from build123d import *

# Parameters (mm, degrees)
F1_DEPTH = 8
F2_W     = 10.1
F2_H     = 10.1
F3_DEPTH = 30
F4_W     = 10.1
F4_H     = 10.1
F5_DEPTH = 33.3550908792
F6_R     = 2


with BuildPart() as f1:
    # F0 (on Right) → F1 (new body, symmetric)
    with BuildSketch(Plane.YZ):
        Polygon((9, -9), (15, -9), (15, 9), (-15, 9), (-15, -9), (-9, -9), (0, -37.9528366029), (16.4139532903, -32.8505531328), align=None)
    extrude(amount=F1_DEPTH, both=True)

    # F2 (on face) → F3 (cut, through all)
    with BuildSketch(Plane(origin=(0, 15, 0), x_dir=(-1, 0, 0), z_dir=(0, 1, 0))):
        Rectangle(F2_W, F2_H)
    extrude(amount=-F3_DEPTH, mode=Mode.SUBTRACT)

    # F4 (on face) → F5 (cut, through all)
    with BuildSketch(Plane(origin=(0, 10.7581183802, -34.608671513), x_dir=(1, 0, 0), z_dir=(0, 0.2968395292, -0.9549273762))):
        with Locations((0, 2.6715557628)):
            Rectangle(F4_W, F4_H)
    extrude(amount=-F5_DEPTH, mode=Mode.SUBTRACT)

    # F6
    f6_edges = [f1.edges().sort_by_distance(p)[0] for p in [
        (0, 15, 9),
        (-8, 0, 9),
        (0, -15, 9),
        (8, 0, 9),
        (-8, 8.206977, -35.401695),
        (-8, 12.706977, -20.925277),
        (-8, 12, -9),
        (-8, 15, 0),
        (-8, -15, 0),
        (-8, -12, -9),
        (-8, -4.5, -23.476418),
        (0, 0, -37.952837),
        (8, -4.5, -23.476418),
        (0, -9, -9),
        (8, 8.206977, -35.401695),
        (8, 12.706977, -20.925277),
        (8, 12, -9),
        (8, 15, 0),
        (8, -15, 0),
        (8, -12, -9),
        (0, 16.413953, -32.850553),
        (0, 9, -9),
        (0, 15, -9),
        (0, -15, -9),
    ]]
    fillet(f6_edges, radius=F6_R)


solid = f1.part
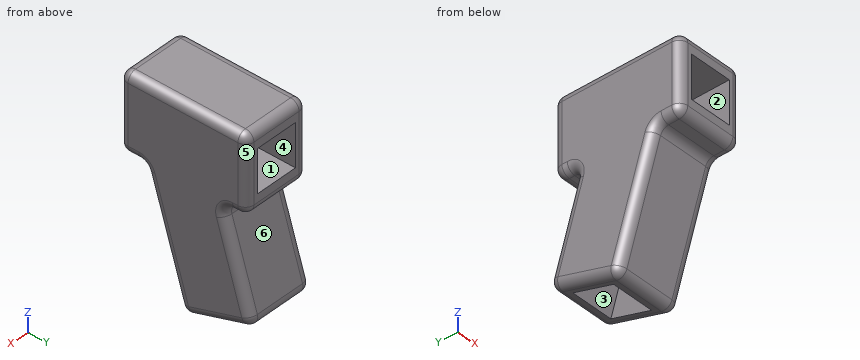
Build history of the part. All positions in model axes, mm. Face numbers are marked on the shaded views. A direction names the side the tool comes from. Coordinates: 2 decimals unless noted, no trailing zeros. Order: outer loops, then holes, each group sorted by start corner. A loop starts at its lowest first (then second) coordinate and runs counter-clockwise, first axis right, second up. Notation, with made-up numbers: (78.5, 6) - (95.5, 6) arc R22 ccw to (95.5, 42) - close; hole circle Ø7 at (-29.75, 18.25). An arc over 180 degrees is marked (long way). Write item = value, one per line. Start each with the question number.
1) Saw through at B-B on z = -0.5. Write the cut outline in (x, y), then the cut area to 3 significant figures.
2) Saw through at A-A on x = -0.5. Write the cut outline in (y, z).
3) Wall check: line 1 along X through (y, z) = (9.5, -26); line 2 along Y through (x, z) = (5.25, 2); line 3 along Y through (x, z) = (1.5, -12). Give the ranges that are in metal, low to high. Write a range as from..to.
4) Saw through at C-C on y = -12. Write the cut outline in (x, z), then the cut area to 3 significant figures.
5) Two-plate mould, pull along X, no slides. Class the marked faces 4, 5 and 6: pulls with the +X half, pulls with the -X half, needs draft (parallel to the pull), parting line crosses it, or undercut.
6) Flat gauge pins, fed straight in: pin 1 Ø8 at (x, y) = (-0.5, 6.5) entering from -Z; pin 2 Ø6 at (x, z) = (5, -9) entering from +Y; pin 3 Ø1.4 at (x, y) = (-2.5, 12.5) entering from -Z. Where does each tip first touch, or does it go through?
7) 3-axis set-ups, long thin cutter, end or side, ignore diameter. For the marked faces 1, 2 and 3: which of +Z, -Z, +X, -X, +Y, -Y reach the whole face in a straight line?
From the geometry:
q1.outline = (-8, -13) arc R2 ccw to (-6, -15) - (-5.05, -15) - (-5.05, 15) - (-6, 15) arc R2 ccw to (-8, 13) - close; (5.05, -15) - (6, -15) arc R2 ccw to (8, -13) - (8, 13) arc R2 ccw to (6, 15) - (5.05, 15) - close
q1.area = 174 mm^2
q2.outline = (-15, -7) arc R2 ccw to (-13, -9) - (-10.47, -9) arc R2 cw to (-8.56, -10.41) - (-0.59, -36.04) arc R2 ccw to (1.91, -37.36) - (3.38, -36.9) - (-6.52, -5.05) - (-15, -5.05) - close; (-15, 5.05) - (15, 5.05) - (15, 7) arc R2 ccw to (13, 9) - (-13, 9) arc R2 ccw to (-15, 7) - close; (4.06, -5.05) - (13.03, -33.9) - (14.5, -33.44) arc R2 ccw to (15.82, -30.94) - (9.81, -11.59) arc R2 cw to (11.72, -9) - (13, -9) arc R2 ccw to (15, -7) - (15, -5.05) - close
q3.line_1 = -8..-5.05, 5.05..8
q3.line_2 = -15..15
q3.line_3 = -8.07..-4.36, 6.22..9.93
q4.outline = (-8, -7) arc R2 ccw to (-6, -9) - (6, -9) arc R2 ccw to (8, -7) - (8, 7) arc R2 ccw to (6, 9) - (-6, 9) arc R2 ccw to (-8, 7) - close; hole (-5.05, -5.05) - (5.05, -5.05) - (5.05, 5.05) - (-5.05, 5.05) - close
q4.area = 183 mm^2
q5.face_4 = undercut
q5.face_5 = pulls with the +X half
q5.face_6 = needs draft
q6.pin_1 = -37.18
q6.pin_2 = 15
q6.pin_3 = -33.9
q7.face_1 = +Y, -Y
q7.face_2 = none
q7.face_3 = -Z
